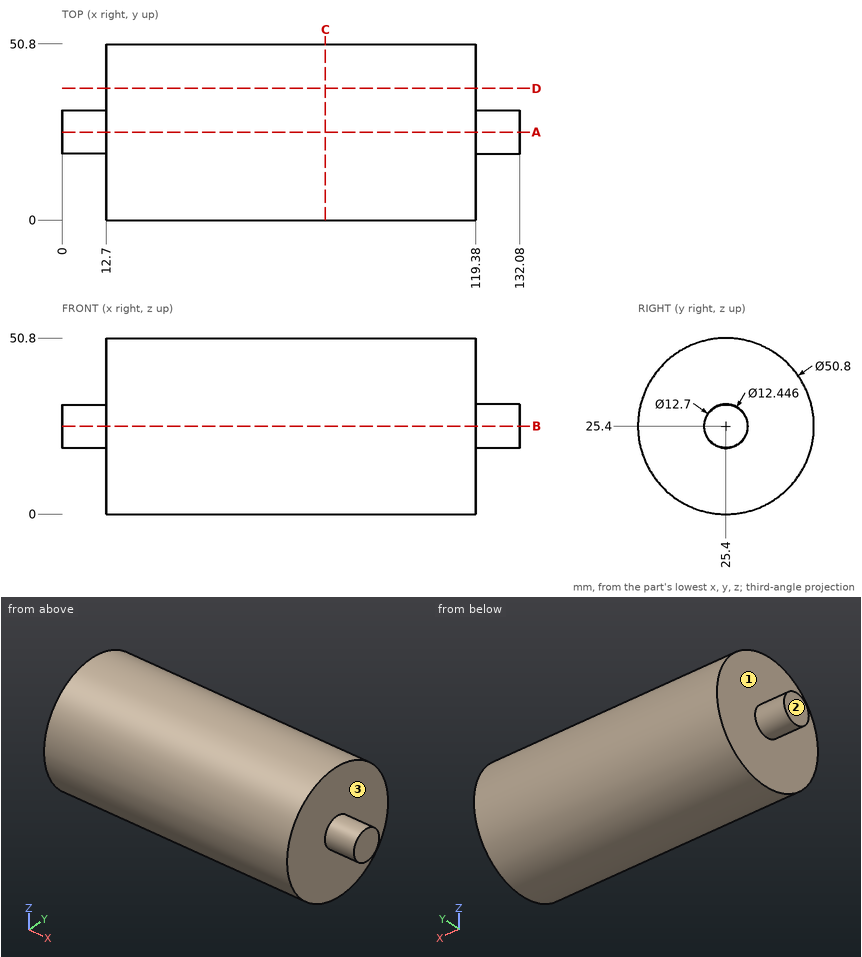
Verification items for this drawing (mm, ordinates from the low corner). A direction names the side the tool comes from. Round coordinates to 2 decimals unless told otherwise and drop trailing zeros. Loops run counter-clockwise (first coordinate to the right, second up) from the corner with the lowest first, then second, coordinate; pieces in that order, holes last. Notation, with made-up numbers: M 75.25,-33.75 L 105.25,-33.75 A17 ccw 105.25,-26.75 Z; hole C -2.75,2 d7. An arc over 180 degrees is marked long. Answer as a JSON object with one key per item and string values.
1. Scan lines: line 1 (X direction, y = 35, z = 36); line 2 (Z direction, x = 68, y = 26.5); line 3 (Z direction, x = 56, y = 28.5). Record each from-to range of solid material in increasing order.
Reply:
{"line 1": "x = 12.7 to 119.38", "line 2": "z = 0.02 to 50.78", "line 3": "z = 0.19 to 50.61"}
2. Access from +Z, -Z, +X, -X, +Y, -Y to the whole of each face (thin tool, end or side, straight path). Record for the marked faces 1, 2 and 3.
Reply:
{"face 1": "-X", "face 2": "+Z, -Z, -X, +Y, -Y", "face 3": "+X"}
3. Section check A-A (y = 25.4). Record the boundary of the cut face in (x, z), plus the area to 3 significant figures.
Reply:
{"outline": "M 0,19.18 L 12.7,19.18 L 12.7,0 L 119.38,0 L 119.38,19.05 L 132.08,19.05 L 132.08,31.75 L 119.38,31.75 L 119.38,50.8 L 12.7,50.8 L 12.7,31.62 L 0,31.62 Z", "area": "5,740 mm²"}
4. Gauge pin test, flat ends, axial feed: P1, Ø10, axis at x = 92.5, z = 13, coming from the +Y side; P2, Ø8, axis at x = 118, z = 35, coming from the -Y side (3 decimals); P3, Ø4, axis at y = 7.5, z = 43.5, coming from the +X side. Record the tip position at first contact, or that the pin passes through.
Reply:
{"P1": "stops at y = 49.7", "P2": "stops at y = 0.625", "P3": "stops at x = 119.38"}
5. Section check D-D (y = 38). Record the boundary of the cut face in (x, z).
Reply:
{"outline": "M 12.7,3.35 L 119.38,3.35 L 119.38,47.45 L 12.7,47.45 Z"}
6. Section check C-C (x = 76). Record the boundary of the cut face in (y, z).
Reply:
{"outline": "C 25.4,25.4 d50.8"}
